Check sheet for the drawn part. Datum: minimum x, y, z corner. Units: mm. Round coordinates to 2 decimals unless told otherwise and drop trailing zeros. Write each loop counter-clockwise with the first axis right and the second up, starting at its lowest first coordinate (ties: lowest second). Pieces come first, ordered by that corner, then holes. Notation, with made-up numbers: (-12, 86) -> (-1, 86) arc R7 cw to (-1, 91) -> close; hole circle Ø10 at (85.25, -26.5). An arc over 180 degrees is marked (long way). Use CSV: the item, a comma, the result in double quotes.
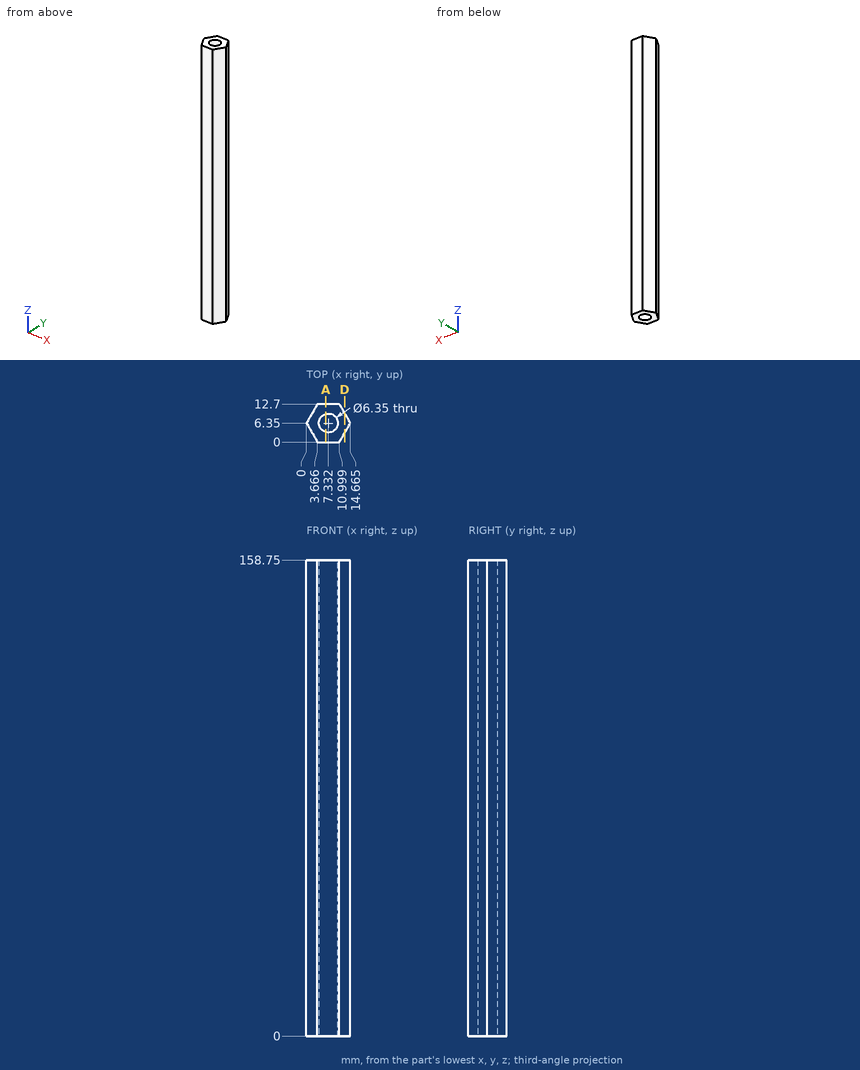
Q1. Section check A-A (x = 6.5). Record the cut outline in (y, z).
Filled in:
outline,"(0, 0) -> (3.29, 0) -> (3.29, 158.75) -> (0, 158.75) -> close; (9.41, 0) -> (12.7, 0) -> (12.7, 158.75) -> (9.41, 158.75) -> close"
Q2. Go/stop test with flat-tipped pins: P1, Ø5, axis at y = 9, z = 38, coming from the +X side; P2, Ø4, axis at x = 3, y = 6.5, coming from the -Z side; P3, Ø3, axis at y = 8, z = 39, coming from the -X side; P4, Ø5.5, axis at x = 7.33, y = 6.35, coming from the +Z side (3 decimals). Record where each tip stops, or that it passes through.
Filled in:
P1,"x = 14.58"
P2,"z = 0"
P3,"x = 0.09"
P4,"through"
Q3. Section check D-D (x = 12.75). Record the cut outline in (y, z), plus the area to 3 significant figures.
Filled in:
outline,"(3.03, 0) -> (9.67, 0) -> (9.67, 158.75) -> (3.03, 158.75) -> close"
area,"1,050 mm²"
Q4. Material ranges on L1, parallel to X at y = 6.35, z = 94.5 (1 decimal); L2, parallel to X at y = 3.75, z = 46 (1 decimal); L3, parallel to Y at x = 9.5, z = 76.5, recorded low to high.
Filled in:
L1,"0 to 4.2, 10.5 to 14.7"
L2,"1.5 to 5.5, 9.2 to 13.2"
L3,"0 to 4.03, 8.67 to 12.7"
